For this review, take the finished solid that the model builds, in its own axes (mm). Face numbers are marked on the shaded views. A direction names the side the tool comes from. Coordinates: 2 decimals unless noted, no trailing zeros. Order: outer loops, then holes, each group sorted by start corner. A loop starts at its lowest first (then second) coordinate and runs counter-clockwise, first axis right, second up. Notation, with made-up numbers: M -10.5,9.5 L 21.5,9.5 A29 ccw 21.5,30.5 Z; hole C 67.5,66 d6. An arc over 180 degrees is marked long. Use CSV: the item, a comma, the result in double quotes.
Autodesk Inventor part; units mm, degrees
ref_plane "Work Plane4" through (0, -3, -40.525) normal (0, 0, 1) x (1, 0, 0)
ref_plane "YZ Plane" through (0, 0, 0) normal (1, 0, 0) x (0, 1, 0)
ref_plane "XZ Plane" through (0, 0, 0) normal (0, 1, 0) x (-1, 0, 0)
sketch "Boceto1" plane through (0, 0, 0) normal (0, 1, 0) x (-1, 0, 0)
  line L0 (0, 0) -> (0, 18)
  line L1 (0, 18) -> (43.0941, 18)
  line L2 (43.0941, 18) -> (43.0941, -103.05)
  line L3 (43.0941, -103.05) -> (0, -103.05)
  line L4 (0, -103.05) -> (0, -81.05)
  line L5 (0, -81.05) -> (34.0941, -81.05)
  line L6 (34.0941, -81.05) -> (34.0941, 0)
  line L7 (34.0941, 0) -> (0, 0)
  dimension "acople_hombro_largo_agujero" = 81.05
  dimension "d1" = 9
  dimension "acople_hombro_grosor_trasero" = 18
  dimension "acople_hombro_ancho_agujero" = 34.0941
  dimension "acople_hombro_grosor_frontal" = 22
extrude "Extrusión1" add sketch "Boceto1" along normal blind 4
sketch "Boceto2" plane through (0, 4, 0) normal (0, 1, 0) x (1, 0, 0)
  line L0 (0, -18) -> (0, 0)
  line L1 (0, 0) -> (-30.5, 0)
  line L2 (-30.5, 0) -> (-30.5, -7.5)
  line L3 (-30.5, -7.5) -> (0, -7.5)
  line L4 (0, -7.5) -> (0, 0)
  point P0 (0, 81.05)
  dimension "d6" = 30.5
  dimension "grosor_seccion_agujero_circular" = 7.5
sketch "Boceto3" plane through (0, 4, 0) normal (0, 1, 0) x (1, 0, 0)
  line L0 (0, 81.05) -> (-30.5, 81.05)
  line L1 (-30.5, 81.05) -> (-30.5, 96.05)
  line L2 (-30.5, 96.05) -> (0, 96.05)
  line L3 (0, 96.05) -> (0, 81.05)
  line L4 (-30.5, 0) -> (-30.5, -7.5)
  point P0 (0, 0)
  dimension "grosor_sección_agujero_servo" = 15
  dimension "d21" = 30.5
extrude "Extrusión2" add sketch "Boceto3" along normal blind 50.5
sketch "Boceto4" plane through (-34.0941, 0, -81.05) normal (0, 0, 1) x (1, 0, 0)
  line L0 (8.5941, 46.5) -> (29.0941, 46.5)
  line L1 (29.0941, 46.5) -> (29.0941, 6)
  line L2 (29.0941, 6) -> (8.5941, 6)
  line L3 (8.5941, 6) -> (8.5941, 46.5)
  line L4 (34.0941, 0) -> (0, 0)
  line L5 (34.0941, 0) -> (34.0941, 54.5)
  line L6 (3.5941, 54.5) -> (34.0941, 54.5)
  line L7 (3.5941, 4) -> (3.5941, 54.5)
  line L8 (0, 0) -> (0, 4)
  circle A0 centre (13.5941, 2.05) radius 1
  circle A1 centre (24.0941, 2.05) radius 1
  circle A2 centre (13.5941, 50.45) radius 1
  circle A3 centre (24.0941, 50.45) radius 1
  line L9 (0, 4) -> (3.5941, 4)
  point P0 (34.0941, 0)
  dimension "d12" = 40.5
  dimension "d13" = 20.5
  dimension "d14" = 2
  dimension "d15" = 3.95
  dimension "d16" = 3.95
  dimension "d17" = 5
  dimension "d18" = 5
  dimension "d19" = 2.05
  dimension "d20" = 5
  dimension "d22" = 30.5
  dimension "d23" = 54.5
  dimension "d24" = 48.4
sketch "Boceto5" plane through (-34.0941, 0, -81.05) normal (0, 0, 1) x (1, 0, 0)
  circle A0 centre (13.5941, 50.45) radius 1
  circle A1 centre (24.0941, 50.45) radius 1
  circle A2 centre (13.5941, 2.05) radius 1
  circle A3 centre (24.0941, 2.05) radius 1
  point P0 (34.0941, 0)
extrude "Extrusión3" cut sketch "Boceto4" against normal up to surface (15 mm away) contours L0 L1 L2 L3
extrude "Extrusión4" cut sketch "Boceto5" against normal up to surface (15 mm away)
extrude "Extrusión5" add sketch "Boceto2" along normal blind 30.5
ref_plane "Plano de trabajo2" through (-25.5, 6, -88.55) normal (0, 1, 0) x (1, 0, 0)
sketch "Boceto6" plane through (0, 0, 0) normal (0, 0, -1) x (-1, 0, 0)
  circle A0 centre (15.25, 16.1) radius 10.9
  line L0 (0, 34.5) -> (30.5, 34.5)
  point P0 (0, 0)
  point P1 (0, 6)
  point P2 (15.25, 34.5)
  dimension "d31" = 10.1
  dimension "d32" = 21.8
extrude "Extrusión6" cut sketch "Boceto6" against normal up to surface (7.5 mm away)
sketch "Boceto7" plane through (0, 4, -96.05) normal (0, 0, -1) x (-1, 0, 0)
  line L0 (0, 0) -> (43.0941, 0)
  line L1 (30.5, 0) -> (30.5, 50.5)
  line L2 (0, 0) -> (30.5, 0)
  line L3 (30.5, 0) -> (30.5, 2)
  line L4 (30.5, 2) -> (0, 2)
  line L5 (0, 2) -> (0, 0)
  line L6 (25.5, 2) -> (5, 2)
  point P0 (0, -4)
extrude "Extrusión7" add sketch "Boceto7" along normal up to surface (7 mm away)
sketch "Sketch13" plane through (0, 0, 0) normal (0, -1, 0) x (1, 0, 0)
  line L0 (0, 0) -> (0, 18)
  line L1 (0, 18) -> (-43.0941, 18)
  line L2 (-43.0941, 18) -> (-43.0941, -103.05)
  line L3 (-43.0941, -103.05) -> (0, -103.05)
  line L4 (0, -103.05) -> (0, -81.05)
  line L5 (0, -81.05) -> (-34.0941, -81.05)
  line L6 (-34.0941, -81.05) -> (-34.0941, 0)
  line L7 (-34.0941, 0) -> (0, 0)
extrude "Extrusion14" add sketch "Sketch13" along normal blind 3
mirror "Mirror2" about plane through (-43.0941, 0, -103.05) normal (-1, 0, 0) of "Extrusión1", "Extrusión2", "Extrusión3", "Extrusión4", "Extrusión5", "Extrusión6", "Extrusión7", "Extrusion14"
sketch "Sketch14" plane through (0, 4, 0) normal (0, 1, 0) x (1, 0, 0)
  line L0 (-30.5, 96.05) -> (-30.5, 103.05)
  line L1 (-30.5, 81.05) -> (-30.5, 103.05)
  line L2 (-55.6882, 96.05) -> (-55.6882, 103.05)
  line L3 (-30.5, 103.05) -> (-55.6882, 103.05)
  line L4 (-55.6882, 103.05) -> (-55.6882, 81.05)
  line L5 (-86.1882, 81.05) -> (-52.0941, 81.05)
  line L6 (-52.0941, 0) -> (-52.0941, 81.05)
  line L7 (-52.0941, 81.05) -> (-52.0941, 0)
  line L8 (-52.0941, 0) -> (-46.0941, 0)
  line L9 (-46.0941, 91.05) -> (-40.0941, 91.05)
  line L10 (-34.0941, 0) -> (-34.0941, 81.05)
  line L11 (-34.0941, 81.05) -> (-30.5, 81.05)
  line L12 (0, 81.05) -> (-34.0941, 81.05)
  line L13 (-34.0941, 0) -> (-34.0941, 81.05)
  line L14 (-30.5, 0) -> (-34.0941, 0)
  line L15 (-34.0941, 0) -> (-30.5, 0)
  line L16 (-30.5, -7.5) -> (-30.5, 0)
  line L17 (-30.5, 0) -> (-30.5, -7.5)
  line L18 (-30.5, -7.5) -> (-40.0941, -7.5)
  line L19 (-40.0941, 91.05) -> (-40.0941, -7.5)
  line L20 (-52.0941, 0) -> (-55.6882, 0)
  line L21 (-52.0941, 0) -> (-86.1882, 0)
  line L22 (-55.6882, 0) -> (-55.6882, -7.5)
  line L23 (-55.6882, -7.5) -> (-46.0941, -7.5)
  line L24 (-46.0941, 91.05) -> (-46.0941, -7.5)
  line L25 (-55.6882, -7.5) -> (-86.1882, -7.5)
  line L26 (-55.6882, -7.5) -> (-55.6882, 0)
  point P0 (0, 0)
  dimension "d65" = 12
  dimension "d66" = 6
  dimension "d68" = 6
  dimension "d69" = 18
extrude "Extrusion15" add sketch "Sketch14" along normal up to surface (2 mm away)
sketch "Sketch15" plane through (0, 4, 0) normal (0, 1, 0) x (1, 0, 0)
  circle A0 centre (-5, -13) radius 2.5
  circle A1 centre (-43.0941, 62.7) radius 2.5
  circle A2 centre (-43.0941, 22.35) radius 2.5
  circle A3 centre (-81.1882, -13) radius 2.5
  line L0 (-46.0941, 91.05) -> (-40.0941, 91.05)
  line L1 (0, -18) -> (-86.1882, -18)
  line L2 (0, -18) -> (0, -7.5)
  line L3 (-86.1882, -18) -> (-86.1882, -7.5)
  line L4 (0, 103.05) -> (-86.1882, 103.05)
  line L5 (-86.1882, 0) -> (-55.6882, 0)
  point P0 (0, 0)
  point P1 (-43.0941, 91.05)
  point P2 (0, 101.05)
  point P3 (-86.1882, 101.05)
  point P4 (-86.1882, 103.05)
  dimension "diametro_tornillo" = 5
  dimension "d73" = 5
  dimension "dist_agujero_trasero_a_lado" = 5
  dimension "d76" = 5
  dimension "d77" = 121.05
  dimension "dist_agujero_central_a_frente" = 40.35
  dimension "d79" = 40.35
  dimension "dist_agujero_trasero_a_frente" = 13
extrude "Extrusion16" cut sketch "Sketch15" along normal mid plane 20
sketch "Sketch16" plane through (0, 4, 0) normal (0, 1, 0) x (1, 0, 0)
  circle A0 centre (-5, -13) radius 2.5
  circle A1 centre (-81.1882, -13) radius 2.5
  circle A2 centre (-81.1882, -13) radius 4.3
  circle A3 centre (-5, -13) radius 2.5
  circle A4 centre (-5, -13) radius 4.3
  point P0 (0, 0)
  dimension "diametro_cabeza_tornillo" = 8.6
extrude "Extrusion17" cut sketch "Sketch16" against normal blind 2
sketch "Sketch17" plane through (-25.5, 6, -81.05) normal (0, 1, 0) x (1, 0, 0)
  circle A0 centre (-17.5941, -18.35) radius 2.5
  circle A1 centre (-17.5941, -18.35) radius 4.3
  circle A2 centre (-17.5941, -58.7) radius 2.5
  circle A3 centre (-17.5941, -58.7) radius 4.3
  circle A4 centre (20.5, -94.05) radius 2.5
  circle A5 centre (20.5, -94.05) radius 4.3
  point P0 (25.5, -81.05)
  dimension "d85" = 8.6
  dimension "d86" = 8.6
extrude "Extrusion18" cut sketch "Sketch17" against normal blind 4 contours A1 | A3
sketch "Sketch18" plane through (-25.5, 6, -81.05) normal (0, 1, 0) x (1, 0, 0)
  circle A0 centre (10.25, 14) radius 2.5
  circle A1 centre (-45.4382, 14) radius 2.5
  circle A2 centre (20.5, -94.05) radius 2.5
  circle A3 centre (-17.5941, -58.7) radius 2.5
  line L0 (20.5, 0) -> (0, 0)
  line L1 (25.5, 22) -> (25.5, 0)
  line L2 (-35.1882, 0) -> (-55.6882, 0)
  line L3 (25.5, 22) -> (-60.6882, 22)
  point P0 (25.5, -81.05)
  point P1 (10.25, 0)
  point P2 (-45.4382, 0)
  point P3 (-60.6882, 20)
  point P4 (-60.6882, 22)
  dimension "dist_agujero_frontal_a_frente" = 8
  dimension "dist_agujero_frontal_a_lateral" = 15.25
extrude "Extrusion19" cut sketch "Sketch18" against normal up to surface (9 mm away) contours A0 | A1
sketch "Sketch19" plane through (-25.5, 6, -81.05) normal (0, 1, 0) x (1, 0, 0)
  circle A0 centre (10.25, 14) radius 2.5
  circle A1 centre (-45.4382, 14) radius 2.5
  circle A2 centre (10.25, 14) radius 4.3
  circle A3 centre (-45.4382, 14) radius 4.3
  circle A4 centre (20.5, -94.05) radius 4.3
  point P0 (25.5, -81.05)
  dimension "d91" = 8.6
  dimension "d98" = 8.6
extrude "Extrusion20" cut sketch "Sketch19" against normal blind 4.5 contours A2 | A3
fillet "Fillet3" radius 3 4 edges at (-86.1882, 1.5, -103.05) (-86.1882, 0.5, 18) (0, 0.5, 18) (0, 1.5, -103.05)
fillet "Fillet3" radius 5 8 edges at (-55.6882, 34.5, 3.75) (-86.1882, 34.5, 3.75) (-86.1882, 54.5, -88.55) (-55.6882, 54.5, -88.55) (-30.5, 54.5, -88.55) (0, 54.5, -88.55) (0, 34.5, 3.75) (-30.5, 34.5, 3.75)
fillet "Fillet3" radius 3 2 edges at (-34.0941, 6, -40.525) (-52.0941, 6, -40.525)
sketch "Sketch20" plane through (0, 4, 0) normal (0, 1, 0) x (1, 0, 0)
  line L0 (-86.1882, -15) -> (-86.1882, -7.5)
  line L1 (0, -15) -> (0, -7.5)
  line L2 (-3, -18) -> (-83.1882, -18)
  line L3 (-5, 0) -> (-25.5, 0)
  point P0 (0, 0)
  dimension "ancho_acople_hombros" = 86.188
sketch "Sketch21" plane through (0, -3, 0) normal (0, 0, -1) x (-1, 0, 0)
  line L0 (3, 0) -> (83.1882, 0)
  line L1 (5, 37.5) -> (25.5, 37.5)
  point P0 (0, 3)
  dimension "altura_acople_circular" = 37.5
ref_plane "Work Plane4" through (0, -3, -40.525) normal (0, 0, 1) x (1, 0, 0)
ref_plane "Work Plane3" through (0, -3, -81.05) normal (0, 0, 1) x (1, 0, 0)
split "Split1" plane through (0, -3, -40.525) removes the side toward (0, 0, -1)
equation "\"d6\" = d21"
equation "\"grosor_sección_agujero_servo\" = 2 * grosor_seccion_agujero_circular"
equation "\"d12\" = largo_servo"
equation "\"d13\" = ancho_servo"
equation "\"d16\" = d15"
equation "\"d18\" = d17"
equation "\"d19\" = -0.5 * d24 - 0.5 * d14 + 0.5 * d23"
equation "\"d20\" = -0.5 * ancho_servo + 0.5 * d22"
equation "\"d29\" = d6"
equation "\"d33\" = d6"
equation "\"d35\" = d6"
equation "\"d66\" = 0.333333 * d69"
equation "\"d68\" = d66"
equation "\"d76\" = dist_agujero_trasero_a_lado"
equation "\"dist_agujero_central_a_frente\" = 0.333333 * d77"
equation "\"d79\" = dist_agujero_central_a_frente"
equation "\"d86\" = d85"
equation "\"d91\" = d98"
equation "\"ancho_hombro\" = 61.05"
equation "\"d104\" = 0.5 * acople_hombro_largo_agujero"
properties part number "Cuerpo - Acople Hombro"
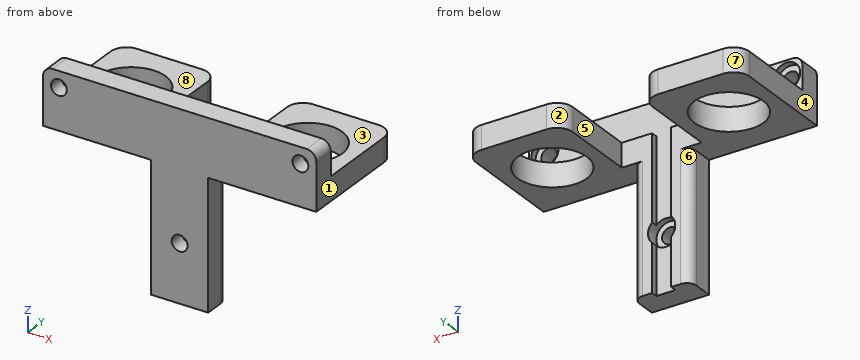
Item 1: Draft analysis for pull direction X (two halves, no side actions). For the marked faces 1, 2 and 3, state which applies: released by +X, released by -X, zero draft, split by the parting line, or undercut.
Solutions:
face 1,"released by +X"
face 2,"undercut"
face 3,"zero draft"
Item 2: Add section C-C on z = 4. State the section outline as (x, y) points, and give its area (3 significant figures).
Solutions:
outline,"M -86.19,-3 L 0,-3 L 0,29.5 A5 ccw -5,34.5 L -25.5,34.5 A5 ccw -30.5,29.5 L -30.5,6 L -40.09,6 L -40.09,4 L -46.09,4 L -46.09,6 L -55.69,6 L -55.69,29.5 A5 ccw -60.69,34.5 L -81.19,34.5 A5 ccw -86.19,29.5 Z; hole C -70.94,16.1 d21.8; hole C -15.25,16.1 d21.8"
area,"1,730 mm^2"
Item 3: Clearance check with flat-ended pins moving along their axes: pin 1 Ø7 at (x, z) = (-81.19, 13) entering from +Y; pin 2 Ø5 at (x, y) = (-24, 11.5) entering from +Z; pin 3 Ø4 at (x, z) = (-5, 13) entering from -Y; pin 4 Ø5 at (x, z) = (-49.5, -6) entering from +Y. State where each tip first meets the part, or that it passes through.
Solutions:
pin 1,"y = 2"
pin 2,"z = 7.5"
pin 3,"through"
pin 4,"y = 6"
Item 4: For the marked faces 4, 5, 6, 7 and 8, list the 3-axis set-ups (+Z, -Z, +X, -X, +Y, -Y) from which the entire face can be reached by the end or side of a thin tool; tool diameter is ignored.
Solutions:
face 4,"+Z, -Z, -X, +Y, -Y"
face 5,"+Z, -Z, +Y"
face 6,"-Z, -X, +Y"
face 7,"+Z, -Z, -X, +Y"
face 8,"+Z, +X, -X, +Y"
Item 5: Add section D-D on y = 16.1. State the section outline as (x, z) points.
Solutions:
outline,"M -86.19,0 L -81.84,0 L -81.84,7.5 L -86.19,7.5 Z; M -60.04,0 L -55.69,0 L -55.69,7.5 L -60.04,7.5 Z; M -30.5,0 L -26.15,0 L -26.15,7.5 L -30.5,7.5 Z; M -4.35,0 L 0,0 L 0,7.5 L -4.35,7.5 Z"
Item 6: Add section B-B on y = 1. State the section outline as (x, z) points (3 decimals), and give its area (3 significant figures).
Solutions:
outline,"M -86.188,0 L -52.094,0 L -52.094,-40.525 L -34.094,-40.525 L -34.094,0 L 0,0 L 0,15 A3 ccw -3,18 L -83.188,18 A3 ccw -86.188,15 Z; hole C -81.188,13 d5; hole C -43.094,-22.35 d5; hole C -5,13 d5"
area,"2,220 mm^2"
Item 7: To check wall thickness, follow line 1 along X through (y, z) = (0, 13); line 2 along X through (y, z) = (-0.75, -22.35); line 3 along Z through (x, y) = (-5, 0.55). State the ranges of each line that lie inside material, in increasing order. Write a range as [from, to].
Solutions:
line 1,"[-86.19, -83.69], [-78.69, -7.5], [-2.5, 0]"
line 2,"[-52.09, -45.59], [-40.59, -34.09]"
line 3,"[0, 10.5], [15.5, 18]"
Item 8: Add section A-A on x = -15.25. State the section outline as (y, z) points, and give its area (3 significant figures).
Solutions:
outline,"M -3,0 L 5.2,0 L 5.2,7.5 L 4,7.5 L 4,18 L -3,18 Z; M 27,0 L 34.5,0 L 34.5,7.5 L 27,7.5 Z"
area,"191 mm^2"
